Autodesk Inventor part; units mm, degrees
ref_plane "YZ Plane" through (0, 0, 0) normal (1, 0, 0) x (0, 1, 0)
ref_plane "XZ Plane" through (0, 0, 0) normal (0, 1, 0) x (-1, 0, 0)
ref_plane "XY Plane" through (0, 0, 0) normal (0, 0, 1) x (1, 0, 0)
sketch "Эскиз1" plane through (0, 0, 0) normal (0, 1, 0) x (-1, 0, 0)
  circle A0 centre (0, 0) radius 46.5
  circle A1 centre (0, 0) radius 38.5
  point P0 (0, 38.5)
  point P1 (0, 46.5)
  dimension "d0" = 93
  dimension "d3" = 8
extrude "Выдавливание1" add sketch "Эскиз1" along normal blind 4
sketch "Эскиз2" plane through (0, 4, 0) normal (0, 1, 0) x (1, 0, 0)
  circle A0 centre (0, 0) radius 46.5
  circle A1 centre (0, 0) radius 42.5
  circle A2 centre (0, 0) radius 46.5
  point P0 (0, -42.5)
  point P1 (0, -46.5)
  point P2 (0, -46.5)
  dimension "d4" = 4
  dimension "d5" = 0
extrude "Выдавливание2" add sketch "Эскиз2" along normal blind 8.5
sketch "Эскиз3" plane through (0, 12.5, 0) normal (0, 1, 0) x (1, 0, 0)
  circle A0 centre (0, 0) radius 46.5
  circle A1 centre (0, 0) radius 50.5
  circle A2 centre (0, 0) radius 46.5
  point P0 (-46.5, 0)
  point P1 (-50.5, 0)
  dimension "d8" = 93
  dimension "d9" = 4
extrude "Выдавливание3" add sketch "Эскиз3" against normal blind 2
properties part number "внешнее кольцо подшипника" material "Стекло"
For this review, take the finished solid that the model builds, in its own axes (mm). A direction names the side the tool comes from. Give positions to 0.01 mm unless a question says otherwise; leave off trailing zeros. Order: outer loops, then holes, each group sorted by start corner. A loop starts at its lowest first (then second) coordinate and runs counter-clockwise, first axis right, second up.
1) Wall thickness on line 1 (Z direction, x = 0, y = 8.75); line 2 (Z direction, x = 0, y = 1.5): over which ranges is each line inside the solid? List them lowest first.
2) Insertion check: pin 1 (3 mm diameter, centred on y = 5.5, z = -13, fed in from -X); pin 2 (4 mm diameter, centred on x = -6, y = 6, fed in from +Z); pin 3 (2 mm diameter, centred on y = 1.5, z = 34.5, fed in from -X). Each pin has a flat end and moves straight along its axis. Give the tip position at first contact, or say it passes through.
3) Take a section at A-A (z = -6). Give the boundary of the cut face in (x, y).
4) Take a section at C-C (y = 2). Give the boundary of the cut face in (x, z), then the cut area to 3 significant figures.
5) For faces 1 (the face through (-33.727, 8.19, -25.861)), 2 (the face through (45, 10.5, 15)), 3 (the face through (17, 0, 35)), list the 3-axis set-ups (+Z, -Z, +X, -X, +Y, -Y) from which the entire face can be reached by the end or side of a thin tool; tool diameter is ignored.
6) The part is to be moulded in two halves that separate along X. For faces 4 (the face through (-23, 12.5, 37)), 5 (the face through (-10.95, 11.51, 49.3)), 6 (the face through (22, 4, 32)), say which applies: released by +X, released by -X, zero draft, split by the parting line, or undercut.
Derived:
1. line 1: z = -46.5 to -42.5, 42.5 to 46.5
1. line 2: z = -46.5 to -38.5, 38.5 to 46.5
2. pin 1: stops at x = -45.06
2. pin 2: stops at z = 46.33
2. pin 3: stops at x = -32.25
3. outline: (-50.14, 10.5) - (-46.11, 10.5) - (-46.11, 0) - (-38.03, 0) - (-38.03, 4) - (-42.07, 4) - (-42.07, 12.5) - (-50.14, 12.5) - close; (38.03, 0) - (46.11, 0) - (46.11, 10.5) - (50.14, 10.5) - (50.14, 12.5) - (42.07, 12.5) - (42.07, 4) - (38.03, 4) - close
4. outline: circle Ø93 at (0, 0); hole circle Ø77 at (0, 0)
4. area: 2,140 mm2
5. face 1: +Y
5. face 2: -Y
5. face 3: +Z, -Z, +X, -X, -Y
6. face 4: zero draft
6. face 5: split by the parting line
6. face 6: undercut
